from build123d import *

# Parameters (mm, degrees)
SKETCH_1_W             = 15
SKETCH_1_H             = 38
SKETCH_1_R             = 2.25
EXTRUDE_1_DEPTH        = 3
FILLET_1_R             = 0.5
CUT_EXTRUDE_1_DEPTH    = 10.5
PATTERN_LINEAR_1_COUNT = 3
PATTERN_LINEAR_1_PITCH = 4.5


with BuildPart() as part:
    # 草图1 → 凸台-拉伸1 (new, symmetric)
    with BuildSketch(Plane.XY):
        Rectangle(SKETCH_1_W, SKETCH_1_H)
        with Locations((0, 14)):
            Circle(SKETCH_1_R, mode=Mode.SUBTRACT)
        with Locations((0, -14)):
            Circle(SKETCH_1_R, mode=Mode.SUBTRACT)
    extrude(amount=EXTRUDE_1_DEPTH, both=True)

    # 圆角1
    fillet_1_edges = [part.edges().sort_by_distance(p)[0] for p in [
        (-7.5, 0, 3),
        (0, -19, 3),
        (7.5, 0, 3),
        (0, -19, -3),
        (-7.5, 0, -3),
        (0, 19, -3),
        (7.5, 0, -3),
        (7.5, -19, 0),
        (-7.5, -19, 0),
        (-7.5, 19, 0),
        (7.5, 19, 0),
        (0, 19, 3),
    ]]
    fillet(fillet_1_edges, radius=FILLET_1_R)

    # 草图2 → 切除-拉伸1 (cut, symmetric)
    with BuildSketch(Plane(origin=(0, 0, 0), x_dir=(1, 0, 0), z_dir=(0, 1, 0))):
        Polygon((-7, 3), (-4.5, 2), (-2, 3), align=None)
    cut_extrude_1 = extrude(amount=CUT_EXTRUDE_1_DEPTH, both=True, mode=Mode.SUBTRACT)

    # 阵列(线性)1: 切除-拉伸1 ×3
    with Locations(*[(i * PATTERN_LINEAR_1_PITCH, 0, 0) for i in range(1, PATTERN_LINEAR_1_COUNT)]):
        add(cut_extrude_1, mode=Mode.SUBTRACT)


solid = part.part
Check sheet for the modelled part. Datum: model origin and axes. Units: mm. A direction names the side the tool comes from. Round coordinates to 2 decimals unless told otherwise and drop trailing zeros. Write each loop counter-clockwise with the first axis right and the second up, starting at its lowest first coordinate (ties: lowest second). Pieces come first, ordered by that corner, then holes. Notation, with made-up numbers: (-11, 75.25) -> (11, 75.25) arc R21 ccw to (11, 108.25) -> close; hole circle Ø3 at (21, -34.75). An arc over 180 degrees is marked (long way). Answer as CSV lines item,"result". Start each with the question number.
1) Tool access check on faces 5 (the flat face through (0, 19, 0)), 6 (the flat face through (-0.1, 10.5, -2.6)). Record the directions out of +Z, -Z, +X, -X, +Y, -Y that give a thin tool (end or side, any length) a straight path to the whole face; none if there is none.
2) Section check C-C on y = 4. Enter the section's corners in (x, z).
3) Release check for a two-part mould opening along X. For faces 1 (the flat face through (7.5, 0, 0)), 2 (the flat face through (-2, -16, -3)), 3 (the flat face through (-3.391, 0.147, -2.444)), 4 (the cylindrical face through (-0.488, -16.196, -0.042)) record: pulls with the +X half, pulls with the -X half, needs draft (parallel to the pull), parting line crosses it, or undercut.
4) Section check A-A on z = 0.2. Enter the section's corners in (x, y).
5) Material ranges on line 1 (Y direction, x = 0, z = 0.5); line 2 (Y direction, x = -0.5, z = -2.5); line 3 (Y direction, x = -0.75, z = -0.9), recorded low to high. Write a range as from..to.
6) Go/stop test with a flat-tipped pin: P1, Ø5, axis at x = 1.5, y = 4, coming from the -Z side. Record where the tip stops, or that it passes through.
7) Section check B-B on y = 14. Enter the section's corners in (x, z), and give its area (3 significant figures).
Found:
1,face 5,"+Z, -Z, +X, -X, +Y"
1,face 6,"-Z"
2,outline,"(-7.5, -2.5) arc R0.5 ccw to (-7, -3) -> (-4.5, -2) -> (-2.25, -2.9) -> (0, -2) -> (2.25, -2.9) -> (4.5, -2) -> (7, -3) arc R0.5 ccw to (7.5, -2.5) -> (7.5, 2.5) arc R0.5 ccw to (7, 3) -> (-7, 3) arc R0.5 ccw to (-7.5, 2.5) -> close"
3,face 1,"pulls with the +X half"
3,face 2,"needs draft"
3,face 3,"undercut"
3,face 4,"undercut"
4,outline,"(-7.5, -18.5) arc R0.5 ccw to (-7, -19) -> (7, -19) arc R0.5 ccw to (7.5, -18.5) -> (7.5, 18.5) arc R0.5 ccw to (7, 19) -> (-7, 19) arc R0.5 ccw to (-7.5, 18.5) -> close; hole circle Ø4.5 at (0, -14); hole circle Ø4.5 at (0, 14)"
5,line 1,"y = -19..-16.25, -11.75..11.75, 16.25..19"
5,line 2,"y = -19..-16.19, -11.81..-10.5, 10.5..11.81, 16.19..19"
5,line 3,"y = -19..-16.12, -11.88..11.88, 16.12..19"
6,P1,"stops at z = -2.9"
7,outline,"(-7.5, -2.5) arc R0.5 ccw to (-7, -3) -> (-2.25, -3) -> (-2.25, 3) -> (-7, 3) arc R0.5 ccw to (-7.5, 2.5) -> close; (2.25, -3) -> (7, -3) arc R0.5 ccw to (7.5, -2.5) -> (7.5, 2.5) arc R0.5 ccw to (7, 3) -> (2.25, 3) -> close"
7,area,"62.8 mm^2"
